from build123d import *

# Parameters (mm, degrees)
CROQUIS1_R              = 50
CROQUIS1_R_2            = 20
SALIENTE_EXTRUIR3_DEPTH = 50
REDONDEO5_R             = 10
REDONDEO6_R             = 7.5


with BuildPart() as part:
    # Croquis1 → Saliente-Extruir3 (new body)
    with BuildSketch(Plane(origin=(0, 0, 0), x_dir=(1, 0, 0), z_dir=(0, 1, 0))):
        with Locations(Location((0, 0, 0), (0, 0, 270))):
            Circle(CROQUIS1_R)
        with Locations(Location((0, 0, 0), (0, 0, 270))):
            Circle(CROQUIS1_R_2, mode=Mode.SUBTRACT)
    extrude(amount=SALIENTE_EXTRUIR3_DEPTH)

    # Redondeo5
    redondeo5_edges = [part.edges().sort_by_distance(p)[0] for p in [
        (0, 0, -50),
        (0, 50, -50),
    ]]
    fillet(redondeo5_edges, radius=REDONDEO5_R)

    # Redondeo6
    redondeo6_edges = [part.edges().sort_by_distance(p)[0] for p in [
        (0, 0, -20),
        (0, 50, -20),
    ]]
    fillet(redondeo6_edges, radius=REDONDEO6_R)


solid = part.part
Here's how the part is built. I have some questions about the finished solid (model axes, mm). Coordinates: 2 decimals unless noted, no trailing zeros. Order: outer loops, then holes, each group sorted by start corner. A loop starts at its lowest first (then second) coordinate and runs counter-clockwise, first axis right, second up.
Item 1: If we section it at C-C on y = 26.5: List the corners of the cut face in (x, z) for me, plus the area to 3 significant figures.
Result sheet:
outline: circle Ø100 at (0, 0); hole circle Ø40 at (0, 0)
area: 6,600 mm2
Item 2: I need wall thicknesses on line 1 (X direction, y = 18, z = 0); line 2 (Z direction, x = -2, y = 2.5); line 3 (Z direction, x = -13, y = 38). Which ranges of each line are inside material? Lowest first, please.
Result sheet:
line 1: x = -50 to -20, 20 to 50
line 2: z = -46.57 to -21.82, 21.82 to 46.57
line 3: z = -48.28 to -15.2, 15.2 to 48.28
Item 3: If we section it at A-A on z = 0: List the corners of the cut face in (x, y) for me, plus the area to 3 significant figures.
Result sheet:
outline: (-50, 10) arc R10 ccw to (-40, 0) - (-27.5, 0) arc R7.5 ccw to (-20, 7.5) - (-20, 42.5) arc R7.5 ccw to (-27.5, 50) - (-40, 50) arc R10 ccw to (-50, 40) - close; (20, 7.5) arc R7.5 ccw to (27.5, 0) - (40, 0) arc R10 ccw to (50, 10) - (50, 40) arc R10 ccw to (40, 50) - (27.5, 50) arc R7.5 ccw to (20, 42.5) - close
area: 2,870 mm2
Item 4: For P1, Ø4, axis at x = 11.5, y = 32, coming from the +Z side; P2, Ø1, axis at x = -13, y = 44, coming from the -Z side; P3, Ø4, axis at x = 10.5, y = 40.5, coming from the +Z side, each with a flat end and sliding along its axis, tell me the tip position at first contact or that it passes through.
Result sheet:
P1: stops at z = 49.09
P2: stops at z = -47.67
P3: stops at z = 49.27
Item 5: If we mould it in two halves opening along X, with no side actions, what happens to faces 1 (the face through (15.02, 24.79, 47.69)), 2 (the face through (-26.1, 0, -9.4)), 3 (the face through (-19.524, 24.755, -4.336))? For each: +X half, -X half, draft (parallel to the pull), parting line (faces both ways), or undercut.
Result sheet:
face 1: parting line
face 2: draft
face 3: undercut
Item 6: If we section it at B-B on x = 0: List the corners of the cut face in (y, z) for me, plus the area to 3 significant figures.
Result sheet:
outline: (0, -40) arc R10 ccw to (10, -50) - (40, -50) arc R10 ccw to (50, -40) - (50, -27.5) arc R7.5 ccw to (42.5, -20) - (7.5, -20) arc R7.5 ccw to (0, -27.5) - close; (0, 27.5) arc R7.5 ccw to (7.5, 20) - (42.5, 20) arc R7.5 ccw to (50, 27.5) - (50, 40) arc R10 ccw to (40, 50) - (10, 50) arc R10 ccw to (0, 40) - close
area: 2,870 mm2
